Check sheet for the modelled part. Datum: model origin and axes. Units: mm. A direction names the side the tool comes from. Round coordinates to 2 decimals unless told otherwise and drop trailing zeros. Order: outer loops, then holes, each group sorted by start corner. A loop starts at its lowest first (then second) coordinate and runs counter-clockwise, first axis right, second up. Notation, with made-up numbers: (83.5, -22.5) -> (124.5, -22.5) arc R19 cw to (124.5, -12.5) -> close; hole circle Ø6 at (3, -26). An arc over 180 degrees is marked (long way). Answer in a Markdown table with one row per item. Add a question column.
1. Draft check along Y on faces 3 (the flat face through (-1, -150.164, 13)), 4 (the flat face through (54, -63.394, 12)), 5 (the flat face through (100, -17, 13)). Enter one of: +Y half, -Y half, draft (parallel to the pull), parting line (faces both ways), or undercut.
2. Sectioned sample at B-B, the plane x = 63. Record the boundary of the cut face in (y, z).
3. Sectioned sample at A-A, the plane y = -102. Record the boundary of the cut face in (x, z), then the cut area to 3 significant figures.
4. Access from +Z, -Z, +X, -X, +Y, -Y to the whole of each face (thin tool, end or side, straight path). Record for faces 1 (the flat face through (96.916, -52, 12)), 2 (the flat face through (-100, -17, 13)).
5. Sectioned sample at C-C, the plane x = -61. Record the boundary of the cut face in (y, z).
6. Sectioned sample at D-D, the plane y = -69.5. Record the boundary of the cut face in (x, z), then the cut area to 3 significant figures.
7. Material ranges on L1, parallel to X at y = -47, z = 20.25; L2, parallel to Y at x = 58, z = 14; L3, parallel to Y at x = -23, z = 15.25, recorded low to high. Write a range as from..to.
```python
from build123d import *

# Parameters (mm, degrees)
SKETCH1_W           = 200
SKETCH1_H           = 240
BOSS_EXTRUDE3_DEPTH = 25
SKETCH3_W           = 87.5
SKETCH3_H           = 110
CUT_EXTRUDE1_DEPTH  = 25
SKETCH4_W           = 200
SKETCH4_H           = 30.164162566
BOSS_EXTRUDE4_DEPTH = 25
CUT_EXTRUDE3_DEPTH  = 40
CUT_EXTRUDE4_DEPTH  = 40
SKETCH8_W           = 72.718372575
SKETCH8_H           = 10
CUT_EXTRUDE5_DEPTH  = 40


with BuildPart() as part:
    # Sketch1 → Boss-Extrude3 (new body)
    with BuildSketch(Plane.XY):
        Rectangle(SKETCH1_W, SKETCH1_H)
    extrude(amount=BOSS_EXTRUDE3_DEPTH)

    # Sketch3 → Cut-Extrude1 (cut)
    with BuildSketch(Plane.XY.offset(25)):
        with Locations((-43.75, -55)):
            Rectangle(SKETCH3_W, SKETCH3_H)
    extrude(amount=-CUT_EXTRUDE1_DEPTH, mode=Mode.SUBTRACT)

    # Sketch4 → Boss-Extrude4 (add)
    with BuildSketch(Plane.XY.offset(25)):
        with Locations((0, -135.082081283)):
            Rectangle(SKETCH4_W, SKETCH4_H)
    extrude(amount=-BOSS_EXTRUDE4_DEPTH)

    # Sketch9 → Cut-Extrude3 (cut)
    with BuildSketch(Plane(origin=(0, 0, 0), x_dir=(-1, 0, 0), z_dir=(0, 0, -1))):
        with BuildLine():
            Line((-91.597538887, -42.469319431), (-91.597538887, -61.749189722))
            ThreePointArc((-91.597538887, -61.749189722), (-94.256831341, -64.408482175), (-96.916123795, -61.749189722))
            Line((-96.916123795, -61.749189722), (-96.916123795, -42.469319431))
            ThreePointArc((-96.916123795, -42.469319431), (-94.256831341, -39.810026977), (-91.597538887, -42.469319431))
        make_face()
    extrude(amount=-CUT_EXTRUDE3_DEPTH, mode=Mode.SUBTRACT)

    # Sketch10 → Cut-Extrude4 (cut)
    with BuildSketch(Plane(origin=(0, 0, 0), x_dir=(-1, 0, 0), z_dir=(0, 0, -1))):
        with BuildLine():
            Line((-75.267088852, -123.445469049), (-41.491938711, -123.445469049))
            ThreePointArc((-41.491938711, -123.445469049), (-38.991938711, -125.945469049), (-41.491938711, -128.445469049))
            Line((-41.491938711, -128.445469049), (-75.267088852, -128.445469049))
            ThreePointArc((-75.267088852, -128.445469049), (-77.767088852, -125.945469049), (-75.267088852, -123.445469049))
        make_face()
    extrude(amount=-CUT_EXTRUDE4_DEPTH, mode=Mode.SUBTRACT)

    # Sketch8 → Cut-Extrude5 (cut)
    with BuildSketch(Plane(origin=(0, 0, 0), x_dir=(-1, 0, 0), z_dir=(0, 0, -1))):
        with Locations((-53.00826824, -68.393983819)):
            Rectangle(SKETCH8_W, SKETCH8_H)
    extrude(amount=-CUT_EXTRUDE5_DEPTH, mode=Mode.SUBTRACT)


solid = part.part
```
Answer key:
| question | item | result |
|---|---|---|
| 1 | face 3 | -Y half |
| 1 | face 4 | undercut |
| 1 | face 5 | draft |
| 2 | outline | (-150.16, 0) -> (-128.45, 0) -> (-128.45, 25) -> (-150.16, 25) -> close; (-123.45, 0) -> (-73.39, 0) -> (-73.39, 25) -> (-123.45, 25) -> close; (-63.39, 0) -> (120, 0) -> (120, 25) -> (-63.39, 25) -> close |
| 3 | outline | (-100, 0) -> (-87.5, 0) -> (-87.5, 25) -> (-100, 25) -> close; (0, 0) -> (100, 0) -> (100, 25) -> (0, 25) -> close |
| 3 | area | 2,810 mm² |
| 4 | face 1 | +Z, -Z |
| 4 | face 2 | +Z, -Z, -X, +Y, -Y |
| 5 | outline | (-150.16, 0) -> (-110, 0) -> (-110, 25) -> (-150.16, 25) -> close; (0, 0) -> (120, 0) -> (120, 25) -> (0, 25) -> close |
| 6 | outline | (-100, 0) -> (-87.5, 0) -> (-87.5, 25) -> (-100, 25) -> close; (0, 0) -> (16.65, 0) -> (16.65, 25) -> (0, 25) -> close; (89.37, 0) -> (100, 0) -> (100, 25) -> (89.37, 25) -> close |
| 6 | area | 995 mm² |
| 7 | L1 | x = -100..-87.5, 0..91.6, 96.92..100 |
| 7 | L2 | y = -150.16..-128.45, -123.45..-73.39, -63.39..120 |
| 7 | L3 | y = -150.16..-110, 0..120 |
